For this review, take the finished solid that the model builds, in its own axes (mm). Coordinates: 2 decimals unless noted, no trailing zeros. Write each loop counter-clockwise with the first axis right and the second up, starting at its lowest first coordinate (ties: lowest second). Pieces come first, ordered by that corner, then holes.
```python
from build123d import *

# Parameters (mm, degrees)
SKETCH_2_W          = 10
SKETCH_2_H          = 0.5
CUT_EXTRUDE_1_DEPTH = 1.06


with BuildPart() as part:
    # 草图1 → 旋转1 (revolve)
    with BuildSketch(Plane(origin=(0, 0, 0), x_dir=(0, 0, -1), z_dir=(1, 0, 0)), mode=Mode.PRIVATE) as revolve_1_sk:
        with BuildLine():
            Line((0, 0), (10.606674091, 0))
            Line((10.606674091, 0), (9.414920498, 1))
            Line((9.414920498, 1), (1.906940731, 1))
            ThreePointArc((1.906940731, 1), (1.817307372, 1.021210009), (1.746685257, 1.08034139))
            Line((1.746685257, 1.08034139), (1.06, 2))
            Line((1.06, 2), (0.606674091, 2))
            ThreePointArc((0.606674091, 2), (0.155005568, 1.044994432), (0, 0))
        make_face()
    revolve(revolve_1_sk.sketch.rotate(Axis((0, 0, 0), (0, 0, -1)), 90), axis=Axis((0, 0, 0), (0, 0, -1)))

    # 草图2 → 切除-拉伸1 (cut)
    with BuildSketch(Plane.XY):
        Rectangle(SKETCH_2_W, SKETCH_2_H)
    extrude(amount=-CUT_EXTRUDE_1_DEPTH, mode=Mode.SUBTRACT)


solid = part.part
```
Q1. Draft analysis for pull direction Y (two halves, no side actions). For faces 1 (the flat face through (0, 0.25, -0.6)), 2 (the cylindrical face through (0, -2, -0.8)), 3 (the cylindrical face through (0, 2, -0.8)), 4 (the flat face through (0, -0.25, -0.6)), state which applies: +Y half, -Y half, draft (parallel to the pull), parting line (faces both ways), or undercut.
Ans:
face 1: undercut
face 2: -Y half
face 3: +Y half
face 4: undercut
Q2. Add section A-A (z = -8). State the section outline as (x, y) points, then the cut area to 3 significant figures.
Ans:
outline: circle Ø2 at (0, 0)
area: 3.14 mm2
Q3. Clearance check with flat-ended pins moving along their axes: pin 1 Ø2 at (x, z) = (-1.5, -2.5) entering from -Y; pin 2 Ø1.5 at (x, z) = (1, -4.5) entering from +Y; pin 3 Ø1 at (x, y) = (1.5, 1.5) entering from -Z. State where each tip first meets the part, or that it passes through.
Ans:
pin 1: stops at y = -0.87
pin 2: stops at y = 0.97
pin 3: stops at z = -1.34
Q4. For probe 1 along Z at (x, y) = (-0.6, -0.75); probe 2 along Y at (x, z) = (-0.15, -8); probe 3 along X at (y, z) = (0.4, -4), list the stretches that pass through material, from the lowest coordinate up.
Ans:
probe 1: z = -9.46 to -0.13
probe 2: y = -0.99 to 0.99
probe 3: x = -0.92 to 0.92
